```python
from build123d import *

# Parameters (mm, degrees)
F0_W     = 25.4
F0_H     = 50.8
F1_DEPTH = 50.8
F2_W     = 19.05
F2_H     = 44.45
F3_DEPTH = 50.8
F5_D     = 5.1054
F7_D     = 5.1054


with BuildPart() as f1:
    # F0 (on Top) → F1 (new body)
    with BuildSketch(Plane.XY):
        with Locations((0.627795, 9.72153)):
            Rectangle(F0_W, F0_H)
    extrude(amount=F1_DEPTH)

    # F2 (on face) → F3 (cut)
    with BuildSketch(Plane.XY.offset(50.8)):
        with Locations((0.627795, 9.72153)):
            Rectangle(F2_W, F2_H)
    extrude(amount=-F3_DEPTH, mode=Mode.SUBTRACT)

    # F5 (through all)
    with Locations(Plane.YZ.offset(13.327795)):
        with Locations((-2.97847, 38.1), (-2.97847, 12.7), (22.42153, 38.1), (22.42153, 12.7)):
            Hole(F5_D / 2)

    # F7 (through all)
    with Locations(Plane(origin=(0, 35.12153, 0), x_dir=(-1, 0, 0), z_dir=(0, 1, 0))):
        with Locations((-0.627795, 38.1), (-0.627795, 12.7)):
            Hole(F7_D / 2)


solid = f1.part
```
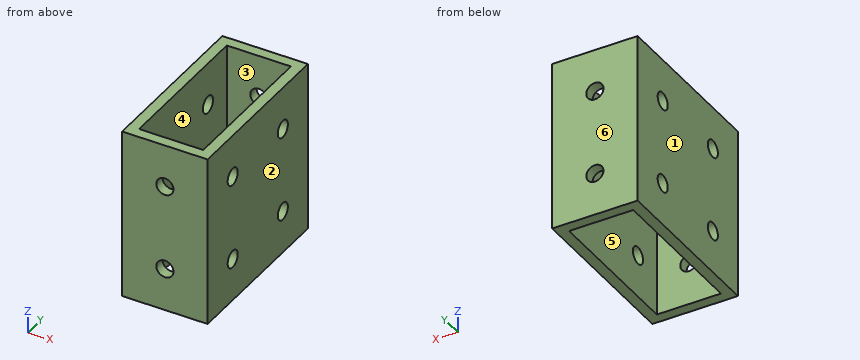
Could you check a few things on this model? Use its own coordinates, in mm. Face numbers are marked on the shaded views. A direction names the side the tool comes from. Round coordinates to 2 decimals unless told otherwise and drop trailing zeros. Loops run counter-clockwise (first coordinate to the right, second up) from the corner with the lowest first, then second, coordinate; pieces in that order, holes last. Notation, with made-up numbers: (89.5, -1) - (124.5, -1) arc R23 cw to (124.5, 15) - close; hole circle Ø5 at (52.25, 32.5). An arc over 180 degrees is marked (long way). Answer in a Markdown table with one row per item. Add a question column.
(1) I'm going to push flat-ended pins straight in: pin 1 (6 mm diameter, centred on x = 0.63, z = 12.7, fed in from -Y); pin 2 (4.5 mm diameter, centred on y = 22.42, z = 12.7, fed in from +X). Where does each tip first touch, or does it pass through?
(2) If we section it at B-B (x = 4.75): Please give me the cut outline in (y, z), plus the area to 3 significant figures.
(3) If we mould it in two halves opening along X, with no side actions, what happens to the marked faces 1, 2, 3 and 4? For each: pulls with the +X half, pulls with the -X half, needs draft (parallel to the pull), parting line crosses it, or undercut.
(4) I need wall thicknesses on line 1 along Y through (x, z) = (6, 29); line 2 along X through (y, z) = (-7, 18); line 3 along X through (y, z) = (32, 38). Which ranges of each line are inside material? Lowest first, please.
(5) If we section it at D-D (x = -10.25): Please give me the cut outline in (y, z), plus the area to 3 significant figures.
(6) If we section it at A-A (y = 0.5): Please give me the cut outline in (x, z).
(7) For the marked faces 5 and 6, which set-ups out of +Z, -Z, +X, -X, +Y, -Y let a thin tool reach every point of the face, with its end or its side?
(8) If we section it at C-C (z = 38.1): State how many separate pieces and enclosed holes the cut face has, plus the area to 3 significant figures.
Model answer:
| question | item | result |
|---|---|---|
| 1 | pin 1 | stops at y = -15.68 |
| 1 | pin 2 | passes through |
| 2 | outline | (-15.68, 0) - (-12.5, 0) - (-12.5, 50.8) - (-15.68, 50.8) - close; (31.95, 0) - (35.12, 0) - (35.12, 50.8) - (31.95, 50.8) - close |
| 2 | area | 323 mm² |
| 3 | face 1 | pulls with the -X half |
| 3 | face 2 | pulls with the +X half |
| 3 | face 3 | undercut |
| 3 | face 4 | undercut |
| 4 | line 1 | y = -15.68 to -12.5, 31.95 to 35.12 |
| 4 | line 2 | x = -12.07 to -8.9, 10.15 to 13.33 |
| 4 | line 3 | x = -12.07 to -1.92, 3.18 to 13.33 |
| 5 | outline | (-15.68, 0) - (35.12, 0) - (35.12, 50.8) - (-15.68, 50.8) - close; hole circle Ø5.11 at (-2.98, 12.7); hole circle Ø5.11 at (-2.98, 38.1); hole circle Ø5.11 at (22.42, 12.7); hole circle Ø5.11 at (22.42, 38.1) |
| 5 | area | 2,500 mm² |
| 6 | outline | (-12.07, 0) - (-8.9, 0) - (-8.9, 50.8) - (-12.07, 50.8) - close; (10.15, 0) - (13.33, 0) - (13.33, 50.8) - (10.15, 50.8) - close |
| 7 | face 5 | +Z, -Z |
| 7 | face 6 | +Z, -Z, +X, -X, +Y |
| 8 | separate pieces | 6 |
| 8 | enclosed holes | 0 |
| 8 | area | 346 mm² |
